Can you work these out from the drawing? Everything is in mm from the part's minimum corner. A direction names the side the tool comes from. Round coordinates to 2 decimals unless told otherwise and drop trailing zeros. Loops run counter-clockwise (first coordinate to the right, second up) from the corner with the lowest first, then second, coordinate; pieces in that order, holes last. Notation, with made-up numbers: M -35.75,64 L 13.25,64 A19 ccw 13.25,75 Z; hole C 66,-22.75 d4. An arc over 180 degrees is marked long. Use a Markdown table: item, result.
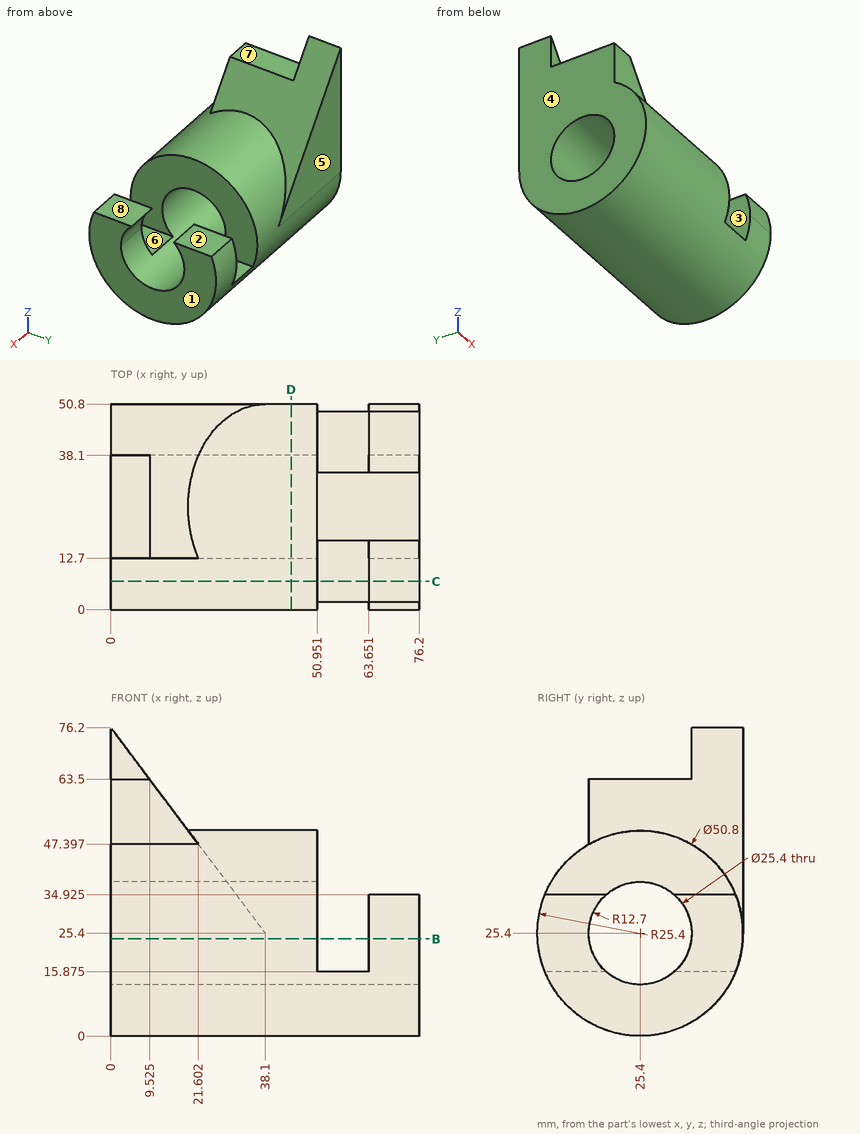
1. I need wall thicknesses on probe 1 along Y at (x, z) = (25.5, 25.4); probe 2 along Z at (x, y) = (24.5, 30.5). Which ranges of each line are inside material? Lowest first, please. Write a range as from..to.
Answer sheet:
| item | result |
|---|---|
| probe 1 | 0..12.7, 38.1..50.8 |
| probe 2 | 0.52..13.77, 37.03..50.28 |
2. Imagine slicing it at B-B, the plane z = 24. Write out the boundary of the cut face in (x, y), then the cut area to 3 significant figures.
Answer sheet:
| item | result |
|---|---|
| outline | M 0,0.04 L 50.95,0.04 L 50.95,12.78 L 0,12.78 Z; M 0,38.02 L 50.95,38.02 L 50.95,50.76 L 0,50.76 Z; M 63.65,0.04 L 76.2,0.04 L 76.2,12.78 L 63.65,12.78 Z; M 63.65,38.02 L 76.2,38.02 L 76.2,50.76 L 63.65,50.76 Z |
| area | 1,620 mm2 |
3. We'd pull the mould along X, two halves only. Please class the marked faces 1, 2 and 3: +X half, -X half, draft (parallel to the pull), parting line (faces both ways), or undercut.
Answer sheet:
| item | result |
|---|---|
| face 1 | +X half |
| face 2 | draft |
| face 3 | undercut |
4. Imagine slicing it at D-D, the plane x = 44.5. Write out the boundary of the cut face in (y, z).
Answer sheet:
| item | result |
|---|---|
| outline | C 25.4,25.4 d50.8; hole C 25.4,25.4 d25.4 |
5. Imagine slicing it at C-C, the plane y = 7. Write out the boundary of the cut face in (x, z) (1 decimal).
Answer sheet:
| item | result |
|---|---|
| outline | M 0,7.9 L 76.2,7.9 L 76.2,34.9 L 63.7,34.9 L 63.7,15.9 L 51,15.9 L 51,42.9 L 0,42.9 Z |
6. Which directions (+Z, -Z, +X, -X, +Y, -Y) give clear straight access to the entire face, cutting with the end or side of a thin tool? Please do the marked faces 4, 5, 6, 7 and 8.
Answer sheet:
| item | result |
|---|---|
| face 4 | +Z, -Z, -X, +Y, -Y |
| face 5 | +Z, -Z, +X, -X, +Y |
| face 6 | +Z, +Y, -Y |
| face 7 | +Z, +X, -X, -Y |
| face 8 | +Z, +X, +Y, -Y |
7. For pin 1 Ø10.5 at (x, y) = (2.5, 23.5) entering from +Z; pin 2 Ø3 at (x, z) = (4, 68.5) entering from -Y; pin 3 Ø10 at (x, y) = (57, 6.5) entering from -Z, each with a flat end and sliding along its axis, tell me the tip position at first contact or that it passes through.
Answer sheet:
| item | result |
|---|---|
| pin 1 | z = 63.5 |
| pin 2 | y = 38.1 |
| pin 3 | z = 4.14 |
